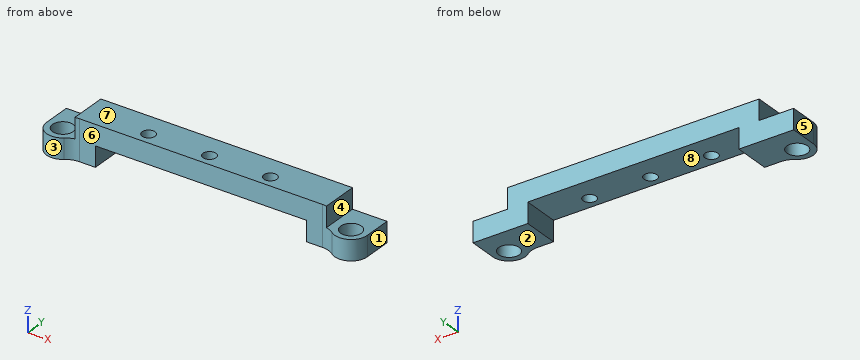
from build123d import *

# Parameters (mm, degrees)
F1_DEPTH = 10.9
F3_DEPTH = 10
F4_R     = 5
F6_D     = 5.1
F9_D     = 3.2


with BuildPart() as f1:
    # F0 (on Front) → F1 (new body)
    with BuildSketch(Plane.XZ):
        Polygon((-26, 0), (0, 0), (0, 5), (-31, 5), (-31, 0), (-39.5, 0), (-39.5, -5), (-26, -5), align=None)
    extrude(amount=F1_DEPTH)

    # F2 (on face) → F3 (cut, through all)
    with BuildSketch(Plane(origin=(0, 0, -5), x_dir=(1, 0, 0), z_dir=(0, 0, -1))):
        with BuildLine():
            ThreePointArc((-39.5, 6.9), (-36.5914129318, 10.7482226823), (-32.0955910939, 9))
            Line((-32.0955910939, 9), (0, 9))
            Line((0, 9), (0, 12.9))
            Line((0, 12.9), (-39.5, 12.9))
            Line((-39.5, 12.9), (-39.5, 6.9))
        make_face()
    extrude(amount=-F3_DEPTH, mode=Mode.SUBTRACT)

    # F4
    f4_edges = [f1.edges().sort_by_distance(p)[0] for p in [
        (-32.095591, -9, -2.5),
    ]]
    fillet(f4_edges, radius=F4_R)

    # F6 (through all)
    with Locations(Plane(origin=(0, 0, -5), x_dir=(1, 0, 0), z_dir=(0, 0, -1))):
        with Locations((-35.5, 6.9)):
            Hole(F6_D / 2)

    # F7: F1 across face


with BuildPart() as f1_1:
    add(f1.part)
    add(f1.part.mirror(Plane(origin=(0, -4.5, 2.5), x_dir=(0, 1, 0), z_dir=(1, 0, 0))))

    # F9 (through all)
    with Locations(Plane(origin=(0, 0, 0), x_dir=(1, 0, 0), z_dir=(0, 0, -1))):
        with Locations((-15, 6), (0, 6), (15, 6)):
            Hole(F9_D / 2)


solid = f1_1.part
Verification items for the finished model (mm, model axes). Face numbers are marked on the shaded views. A direction names the side the tool comes from. Coordinates: 2 decimals unless noted, no trailing zeros. Loops run counter-clockwise (first coordinate to the right, second up) from the corner with the lowest first, then second, coordinate; pieces in that order, holes last. Notation, with made-up numbers: (-10, 29.25) -> (11, 29.25) arc R14 cw to (11, 53.25) -> close; hole circle Ø10 at (-33.5, 36.25). An arc over 180 degrees is marked (long way). Write each question's results on one line, items separated by ' | '.
Item 1: Mould release check, pull along X, two halves, no side actions. Record for the marked faces 1, 2 and 3: +X half, -X half, draft (parallel to the pull), parting line (faces both ways), or undercut.
Found:
face 1: +X half | face 2: draft | face 3: undercut
Item 2: Section check C-C, the plane y = -6. Count the separate pieces of the cut face and the enclosed holes in it, plus the area to 3 significant figures.
Found:
separate pieces: 6 | enclosed holes: 0 | area: 349 mm2
Item 3: Section check A-A, the plane x = -15. Enter the section's corners in (y, z).
Found:
outline: (-9, 0) -> (-7.6, 0) -> (-7.6, 5) -> (-9, 5) -> close; (-4.4, 0) -> (0, 0) -> (0, 5) -> (-4.4, 5) -> close
Item 4: Tool access check on the marked faces 4, 5, 6, 7 and 8. Record the directions out of +Z, -Z, +X, -X, +Y, -Y that give a thin tool (end or side, any length) a straight path to the whole face; none if there is none.
Found:
face 4: +Z, +X, +Y, -Y | face 5: +Z, -Z, -X, +Y, -Y | face 6: +Z, -Z, -Y | face 7: +Z, +X, -X, +Y, -Y | face 8: -Z, +Y, -Y
Item 5: Section check D-D, the plane z = 2.25. Enter the section's corners in (x, y), plus the area to 3 significant figures.
Found:
outline: (-31, -9.11) arc R5 cw to (-29.97, -9) -> (29.97, -9) arc R5 cw to (31, -9.11) -> (31, 0) -> (-31, 0) -> close; hole circle Ø3.2 at (-15, -6); hole circle Ø3.2 at (0, -6); hole circle Ø3.2 at (15, -6) | area: 534 mm2
Item 6: Material ranges on L1, parallel to X at y = -6, z = 3.75; L2, parallel to Y at x = 0, z = 2.7; L3, parallel to Y at x = -35.5, z = -3.7, recorded low to high.
Found:
L1: x = -31 to -16.6, -13.4 to -1.6, 1.6 to 13.4, 16.6 to 31 | L2: y = -9 to -7.6, -4.4 to 0 | L3: y = -10.9 to -9.45, -4.35 to 0
Item 7: Gauge pin test, flat ends, axial feed: pin 1 (2.5 mm diameter, centred on x = 7, y = -3.5, fed in from -Z); pin 2 (1.5 mm diameter, centred on y = -6.5, z = 1.5, fed in from +X); pin 3 (4 mm diameter, centred on x = 33.5, y = -5, fed in from +Z). Record the tip position at first contact, or that the pin passes through.
Found:
pin 1: stops at z = 0 | pin 2: stops at x = 31 | pin 3: stops at z = 0
Item 8: Section check B-B, the plane z = -2.5. Enter the section's corners in (x, y).
Found:
outline: (-39.5, -6.9) arc R4 ccw to (-33.04, -10.06) arc R5 cw to (-29.97, -9) -> (-26, -9) -> (-26, 0) -> (-39.5, 0) -> close; (26, -9) -> (29.97, -9) arc R5 cw to (33.04, -10.06) arc R4 ccw to (39.5, -6.9) -> (39.5, 0) -> (26, 0) -> close; hole circle Ø5.1 at (-35.5, -6.9); hole circle Ø5.1 at (35.5, -6.9)
